Print and shaded views of the part. All mm, measured from the part's lowest x, y and z. A direction names the side the tool comes from. Coordinates: 2 decimals unless noted, no trailing zeros. Order: outer loops, then holes, each group sorted by start corner. A loop starts at its lowest first (then second) coordinate and runs counter-clockwise, first axis right, second up. Notation, with made-up numbers: (87, 63) -> (130, 63) arc R13 cw to (130, 77) -> close; hole circle Ø4 at (-35, 59.5). An arc over 180 degrees is marked (long way). Return JSON: item names as keys, results as strings. Group by question number.
1) Cut at B-B (x = 13.5). Write the cut outline in (y, z), and give its area (3 significant figures).
2) Pull direction Z, two halves, no side cores. Call the marked faces 1, 2 and 3: +Z half, -Z half, draft (parallel to the pull), parting line (faces both ways), or undercut.
3) Cut at C-C (z = 33). Write the cut outline in (x, y), and give its area (3 significant figures).
4) Cut at D-D (z = 23). Write the cut outline in (x, y), and give its area (3 significant figures).
5) Which spindle directions (+Z, -Z, +X, -X, +Y, -Y) get a long thin tool onto all of the face, cutting with end or side? Do the marked faces 4, 5 and 6. Say none if no direction does.
6) Flat gauge pins, fed straight in: pin 1 (1.5 mm diameter, centred on x = 6.5, z = 17, fed in from -Y); pin 2 (1.3 mm diameter, centred on x = 17.5, z = 34, fed in from -Y); pin 3 (5 mm diameter, centred on x = 9.5, z = 9, fed in from -Y). Where does each tip first touch, or does it go through?
7) Probe line 1 (Z direction, x = 18.5, y = 7.5); line 2 (Z direction, x = 12.5, y = 11.5); line 3 (Y direction, x = 13.5, z = 27.5). List the from-to ranges inside material, lowest first.
8) Cut at A-A (y = 4). Write the cut outline in (x, z), and give its area (3 significant figures).
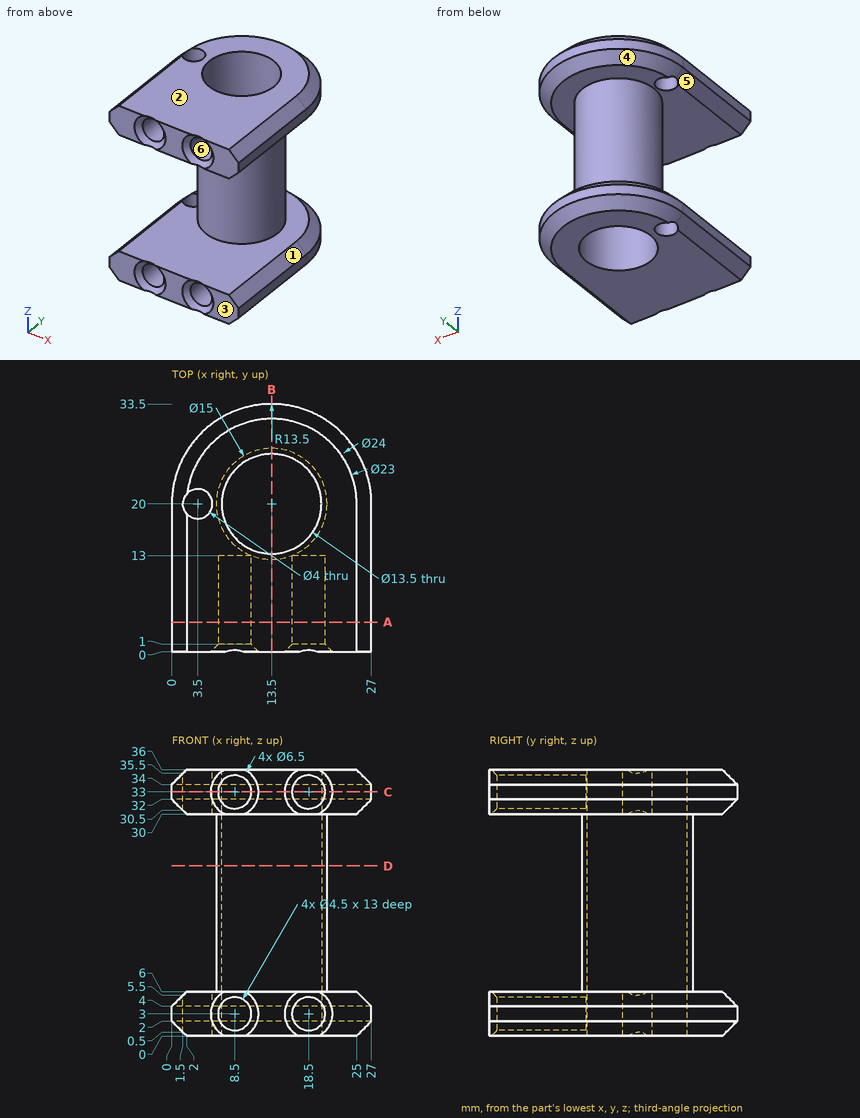
Answers below:
{
 "1": {"outline": "(0, 0) -> (13.25, 0) -> (13.25, 36) -> (0, 36) -> (0, 30) -> (12.5, 30) -> (12.5, 6) -> (0, 6) -> close; (26.75, 0) -> (31.5, 0) -> (33.5, 2) -> (33.5, 4) -> (31.5, 6) -> (27.5, 6) -> (27.5, 30) -> (31.5, 30) -> (33.5, 32) -> (33.5, 34) -> (31.5, 36) -> (26.75, 36) -> close", "area": "268 mm^2"},
 "2": {"face 1": "undercut", "face 2": "+Z half", "face 3": "draft"},
 "3": {"outline": "(0, 0) -> (5.25, 0) -> (6.25, 1) -> (6.25, 13) -> (10.75, 13) -> (10.75, 1) -> (11.75, 0) -> (15.25, 0) -> (16.25, 1) -> (16.25, 13) -> (20.75, 13) -> (20.75, 1) -> (21.75, 0) -> (27, 0) -> (27, 20) arc R13.5 ccw to (0, 20) -> close; hole circle Ø4 at (3.5, 20); hole circle Ø13.5 at (13.5, 20)", "area": "552 mm^2"},
 "4": {"outline": "circle Ø15 at (13.5, 20); hole circle Ø13.5 at (13.5, 20)", "area": "33.6 mm^2"},
 "5": {"face 4": "+Y", "face 5": "-X, +Y, -Y", "face 6": "-Y"},
 "6": {"pin 1": "stops at y = 15.85", "pin 2": "stops at y = 13", "pin 3": "stops at y = 12.65"},
 "7": {"line 1": "z = 0 to 0.75, 5.25 to 6, 30 to 30.75, 35.25 to 36", "line 2": "z = 0 to 6, 30 to 36", "line 3": "y = 12.5 to 13.25, 26.75 to 27.5"},
 "8": {"outline": "(0, 2) -> (2, 0) -> (25, 0) -> (27, 2) -> (27, 4) -> (25, 6) -> (2, 6) -> (0, 4) -> close; (0, 32) -> (2, 30) -> (25, 30) -> (27, 32) -> (27, 34) -> (25, 36) -> (2, 36) -> (0, 34) -> close; hole circle Ø4.5 at (8.5, 3); hole circle Ø4.5 at (8.5, 33); hole circle Ø4.5 at (18.5, 3); hole circle Ø4.5 at (18.5, 33)", "area": "244 mm^2"}
}
